Work out the finished part from the listing and answer in its coordinate system (mm). A direction names the side the tool comes from. Coordinates: 2 decimals unless noted, no trailing zeros. Loops run counter-clockwise (first coordinate to the right, second up) from the corner with the lowest first, then second, coordinate; pieces in that order, holes last. Notation, with made-up numbers: (45.25, 74) -> (56.25, 74) arc R21 ccw to (56.25, 111) -> close; hole circle Ø2 at (23.5, -14). An arc over 180 degrees is marked (long way). Use a Markdown table: item, result. Add a question column.
Autodesk Inventor part; units mm, degrees
ref_plane "YZ Plane" through (0, 0, 0) normal (1, 0, 0) x (0, 1, 0)
ref_plane "XZ Plane" through (0, 0, 0) normal (0, 1, 0) x (-1, 0, 0)
ref_plane "XY Plane" through (0, 0, 0) normal (0, 0, 1) x (1, 0, 0)
sketch "Sketch1" plane through (0, 0, 0) normal (0, 1, 0) x (-1, 0, 0)
  line L0 (50, -10) -> (-50, -10)
  line L1 (-50, -10) -> (-50, 10)
  line L2 (-50, 10) -> (50, 10)
  line L3 (50, 10) -> (50, -10)
  line L4 (50, -10) -> (-50, 10) construction
  line L5 (-50, -10) -> (50, 10) construction
  line L6 (48, -8) -> (-48, -8)
  line L7 (-48, -8) -> (-48, 8)
  line L8 (-48, 8) -> (48, 8)
  line L9 (48, 8) -> (48, -8)
  line L10 (48, -8) -> (-48, 8) construction
  line L11 (-48, -8) -> (48, 8) construction
  point P0 (0, 0)
  dimension "d2" = 100
  dimension "d3" = 20
  dimension "d4" = 96
  dimension "d5" = 16
extrude "Extrusion1" add sketch "Sketch1" along normal blind 348
sketch "Sketch2" plane through (-50, 0, 10) normal (0, 0, 1) x (1, 0, 0)
  circle A0 centre (10, 40) radius 2.75
  circle A1 centre (90, 40) radius 2.75
  circle A2 centre (10, 308) radius 2.75
  circle A3 centre (90, 308) radius 2.75
  line L0 (0, 348) -> (100, 348)
  line L1 (0, 0) -> (0, 348)
  line L2 (100, 0) -> (100, 348)
  line L3 (100, 0) -> (0, 0)
  point P0 (50, 0)
  dimension "d8" = 5.5
  dimension "d9" = 5.5
  dimension "d10" = 5.5
  dimension "d11" = 5.5
  dimension "d12" = 40
  dimension "d13" = 10
  dimension "d14" = 10
  dimension "d15" = 40
  dimension "d16" = 40
  dimension "d17" = 10
  dimension "d18" = 40
  dimension "d19" = 10
extrude "Extrusion2" cut sketch "Sketch2" against normal through all contours A0 | A1 | A2 | A3
sketch "Sketch3" plane through (-50, 0, -10) normal (-1, 0, 0) x (0, 0, 1)
  circle A0 centre (10, 16) radius 2.75
  line L0 (10, 16) -> (10, 0) construction
  line L1 (0, 0) -> (0, 348)
  circle A1 centre (10, 32) radius 2.75
  circle A2 centre (10, 48) radius 2.75
  circle A3 centre (10, 64) radius 2.75
  circle A4 centre (10, 80) radius 2.75
  circle A5 centre (10, 96) radius 2.75
  circle A6 centre (10, 112) radius 2.75
  circle A7 centre (10, 128) radius 2.75
  circle A8 centre (10, 144) radius 2.75
  circle A9 centre (10, 160) radius 2.75
  circle A10 centre (10, 176) radius 2.75
  circle A11 centre (10, 192) radius 2.75
  circle A12 centre (10, 208) radius 2.75
  circle A13 centre (10, 224) radius 2.75
  circle A14 centre (10, 240) radius 2.75
  circle A15 centre (10, 256) radius 2.75
  circle A16 centre (10, 272) radius 2.75
  circle A17 centre (10, 288) radius 2.75
  circle A18 centre (10, 304) radius 2.75
  circle A19 centre (10, 320) radius 2.75
  circle A20 centre (10, 336) radius 2.75
  circle A21 centre (10, 352) radius 2.75
  circle A22 centre (10, 368) radius 2.75
  circle A23 centre (10, 384) radius 2.75
  circle A24 centre (10, 400) radius 2.75
  circle A25 centre (10, 416) radius 2.75
  circle A26 centre (10, 432) radius 2.75
  dimension "d22" = 5.5
  dimension "d23" = 16
  dimension "d26" = 16
extrude "Extrusion3" cut sketch "Sketch3" against normal through all
sketch "Sketch4" plane through (-50, 0, 10) normal (0, 0, 1) x (1, 0, 0)
  line L0 (0, 348) -> (100, 348)
  circle A0 centre (87, 348) radius 7.5
  line L1 (2, 348) -> (98, 348)
  line L2 (100, 0) -> (0, 0)
  circle A1 centre (87, 0) radius 7.5
  line L3 (100, 0) -> (100, 348)
  point P0 (50, 0)
  dimension "d33" = 15
  dimension "d35" = 15
  dimension "d36" = 13
  dimension "d37" = 13
extrude "Extrusion4" cut sketch "Sketch4" against normal blind 10
sketch "Sketch5" plane through (-50, 0, 10) normal (0, 0, 1) x (1, 0, 0)
  circle A0 centre (50, 50) radius 30
  line L0 (79.5, 0) -> (0, 0)
  line L1 (100, 0) -> (100, 348)
  line L2 (0, 0) -> (0, 348)
  line L3 (0, 174) -> (100, 174)
  line L4 (0, 348) -> (79.5, 348)
  circle A1 centre (50, 130) radius 30
  circle A2 centre (50, 298) radius 30
  circle A3 centre (50, 218) radius 30
  point P0 (50, 0)
  dimension "d40" = 60
  dimension "d41" = 50
  dimension "d42" = 50
  dimension "d50" = 174
  dimension "d53" = 80
extrude "Extrusion5" cut sketch "Sketch5" against normal blind 50
properties part number "Mid" material "Aluminum 6061"
Item 1: Section A-A (x = -34) is taken. Determine the outline of the cut face in (y, z), then the cut area to 3 significant figures.
Item 2: Section B-B (y = 230.5) is taken. Determine the outline of the cut face in (x, z), then the cut area to 3 significant figures.
Item 3: Given pin 1 (4.5 mm diameter, centred on x = -40, y = 40, fed in from +Z), flat-ended and moving along its own axis, determine where the tip first touches the part or whether it passes through.
Item 4: For faces 4 (the face through (-49.014, 237.315, -0.596)), 5 (the face through (36.84, 340.5, 9.01)), 6 (the face through (-1, 172, -8)), determine the directions among +Z, -Z, +X, -X, +Y, -Y from which every point of the face is accessible in a straight line to the end or side of a thin tool.
Item 5: For a pull along X with two mould halves and no side action, classify faces 1 (the face through (50, 172, 0)), 2 (the face through (-42.027, 41.859, -8.986)), 3 (the face through (-49.014, 77.315, -0.596)) as +X half, -X half, draft (parallel to the pull), parting line (faces both ways), or undercut.
Item 6: Section C-C (x = 13) is taken. Count the separate pieces of the cut face and the enclosed holes in it, then the cut area to 3 significant figures.
Item 7: Find the intervals of material crossed by probe 1 along Y at (x, z) = (-40, 9); probe 2 along Z at (x, y) = (-27, 147.5); probe 3 along X at (y, z) = (308, 9.55), in increasing order.
Output:
| question | item | result |
|---|---|---|
| 1 | outline | (0, -10) -> (348, -10) -> (348, -8) -> (0, -8) -> close; (0, 8) -> (348, 8) -> (348, 10) -> (0, 10) -> close |
| 1 | area | 1,390 mm2 |
| 2 | outline | (-50, -10) -> (-27.27, -10) -> (-27.27, -8) -> (-48, -8) -> (-48, 8) -> (-27.27, 8) -> (-27.27, 10) -> (-50, 10) -> close; (27.27, -10) -> (50, -10) -> (50, 10) -> (27.27, 10) -> (27.27, 8) -> (48, 8) -> (48, -8) -> (27.27, -8) -> close |
| 2 | area | 246 mm2 |
| 3 | pin 1 | passes through |
| 4 | face 4 | +X, -X |
| 4 | face 5 | +Z, +Y |
| 4 | face 6 | +Y, -Y |
| 5 | face 1 | +X half |
| 5 | face 2 | undercut |
| 5 | face 3 | draft |
| 6 | separate pieces | 10 |
| 6 | enclosed holes | 0 |
| 6 | area | 527 mm2 |
| 7 | probe 1 | y = 0 to 37.25, 42.75 to 305.25, 310.75 to 348 |
| 7 | probe 2 | z = -10 to -8, 8 to 10 |
| 7 | probe 3 | x = -50 to -42.75, -37.25 to -28.28, 28.28 to 37.25, 42.75 to 50 |
